The listing builds one solid part. Answer for the finished solid, in the listing's coordinates (mm). Face numbers are marked on the shaded views. Give positions to 0.01 mm unless a question says otherwise; leave off trailing zeros. Order: outer loops, then holes, each group sorted by start corner. A loop starts at its lowest first (then second) coordinate and runs counter-clockwise, first axis right, second up. Notation, with made-up numbers: (-23.5, -34) - (32.5, -34) arc R29 ccw to (32.5, 5) - close; hole circle Ø5 at (2, 15). An arc over 180 degrees is marked (long way). Write each question's results on one line, items separated by ' | '. Start each with the question number.
1. Find the intervals of material crossed by L1, parallel to Y at x = 58.5, z = 11; L2, parallel to Y at x = -49.5, z = 2.5; L3, parallel to Y at x = 102, z = 11.75, in increasing order.
2. Section A-A (x = 60) is taken. Give the vertices of the cut face in (y, z).
3. Section B-B (y = -54) is taken. Give the vertices of the cut face in (x, z).
4. Section D-D (y = -80) is taken. Give the vertices of the cut face in (x, z), and give its area (3 significant figures).
5. Flat-ended cylindrical pins translate along their axes: pin 1 (1 mm diameter, centred on y = -20.5, z = 13, fed in from -X); pin 2 (5 mm diameter, centred on x = 16.02, y = -34.5, fed in from +Z); pin 3 (8 mm diameter, centred on x = 33.5, z = 22.5, fed in from -Y); pin 4 (4 mm diameter, centred on x = 68.5, z = 20, fed in from -Y). Find the tip coordinate at first contact, or state that the pin passes through.
6. Determine the mould class of the marked faces 1, 2 and 3 for opening direction X: released by +X, released by -X, zero draft, split by the parting line, or undercut.
7. Section C-C (z = 5.5) is taken. Give the vertices of the cut face in (x, y) (3 decimals), and give its area (3 significant figures).
from build123d import *

# Parameters (mm, degrees)
F0_R     = 29.182002
F1_DEPTH = 25.4
F3_D     = 6.35


with BuildPart() as f1:
    # F0 (on Top) → F1 (new body)
    with BuildSketch(Plane.XY):
        Polygon((161.236733, 0), (-85.090756, 0), (-86.466879, -91.804653), align=None)
        with Locations((-42.430699, -39.840698)):
            Circle(F0_R, mode=Mode.SUBTRACT)
    extrude(amount=F1_DEPTH)

    # F3 (through all)
    with Locations(Plane.XY.offset(25.4)):
        with Locations((20.763323, -17.923191), (16.023301, -34.498475), (59.114777, -18.968618)):
            Hole(F3_D / 2)


solid = f1.part
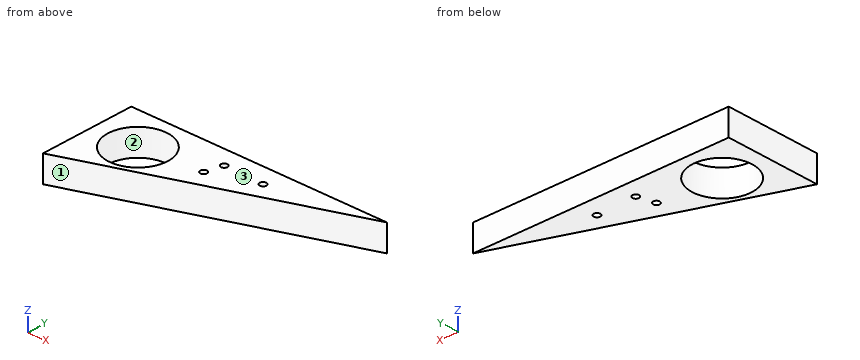
Reported:
1) L1: -38.08 to -22.08, -15.85 to 0 | L2: -78.1 to -68.15, -11.53 to 0 | L3: -21.95 to 0
2) outline: (-37.52, 0) - (-22.02, 0) - (-22.02, 25.4) - (-37.52, 25.4) - close; (-15.92, 0) - (0, 0) - (0, 25.4) - (-15.92, 25.4) - close
3) outline: (-85.9, 0) - (-67.95, 0) - (-67.95, 25.4) - (-85.9, 25.4) - close; (-16.91, 0) - (15.54, 0) - (15.54, 25.4) - (-16.91, 25.4) - close
4) outline: (-86.29, 0) - (-54.62, 0) - (-54.62, 25.4) - (-86.29, 25.4) - close | area: 805 mm²
5) pin 1: x = -85.41 | pin 2: through | pin 3: y = -48.82 | pin 4: y = -35.11
6) face 1: released by +X | face 2: undercut | face 3: zero draft
7) outline: (-86.467, -91.805) - (161.237, 0) - (-85.091, 0) - close; hole circle Ø58.364 at (-42.431, -39.841); hole circle Ø6.35 at (16.023, -34.498); hole circle Ø6.35 at (20.763, -17.923); hole circle Ø6.35 at (59.115, -18.969) | area: 8,540 mm²
